```python
from build123d import *

# Parameters (mm, degrees)
SKETCH_1_R               = 10
EXTRUDE_1_DEPTH          = 4
SKETCH_3_R               = 3
CUT_EXTRUDE_1_DEPTH      = 15.696938457
SKETCH_5_R               = 1
CUT_EXTRUDE_2_DEPTH      = 15.696938457
PATTERN_CIRCULAR_1_COUNT = 8
SKETCH_6_R               = 3.5
SKETCH_6_R_2             = 3
EXTRUDE_3_DEPTH          = 0.5
FILLET_3_R               = 0.2
EXTRUDE_START            = -1.6
SKETCH_7_R               = 3.5
SKETCH_7_R_2             = 1.25
EXTRUDE_4_DEPTH          = 1.6


with BuildPart() as part:
    # Sketch 1 → Extrude 1 (new body)
    with BuildSketch(Plane(origin=(0, 0, 0), x_dir=(0, 0, -1), z_dir=(1, 0, 0))):
        Circle(SKETCH_1_R)
    extrude(amount=EXTRUDE_1_DEPTH)

    # Sketch 3 → Cut-Extrude 1 (cut, through all)
    with BuildSketch(Plane(origin=(4, 0, 0), x_dir=(0, 0, -1), z_dir=(1, 0, 0))):
        Circle(SKETCH_3_R)
    extrude(amount=-CUT_EXTRUDE_1_DEPTH, mode=Mode.SUBTRACT)

    # Sketch 5 → Cut-Extrude 2 (cut, through all)
    with BuildSketch(Plane.ZY):
        with Locations((0, 7)):
            Circle(SKETCH_5_R)
    cut_extrude_2 = extrude(amount=-CUT_EXTRUDE_2_DEPTH, mode=Mode.SUBTRACT)

    # Pattern Circular 1: Cut-Extrude 2 ×8 about axis
    pattern_circular_1_axis = Axis((0, 0, 0), (1, 0, 0))
    for i in range(1, PATTERN_CIRCULAR_1_COUNT):
        add(cut_extrude_2.rotate(pattern_circular_1_axis, i * 360 / PATTERN_CIRCULAR_1_COUNT), mode=Mode.SUBTRACT)

    # Sketch 6 → Extrude 3 (add)
    with BuildSketch(Plane.ZY):
        with Locations(Location((0, 0, 0), (0, 0, 180))):
            Circle(SKETCH_6_R)
        with Locations(Location((0, 0, 0), (0, 0, 180))):
            Circle(SKETCH_6_R_2, mode=Mode.SUBTRACT)
    extrude(amount=EXTRUDE_3_DEPTH)

    # Fillet 3
    fillet_3_edges = [part.edges().sort_by_distance(p)[0] for p in [
        (-0.5, 0, 3.5),
        (-0.5, 0, 3),
    ]]
    fillet(fillet_3_edges, radius=FILLET_3_R)

    # Sketch 7 → Extrude 4 (add)
    with BuildSketch(Plane.ZY.offset(EXTRUDE_START)):
        with Locations(Location((0, 0, 0), (0, 0, 180))):
            Circle(SKETCH_7_R)
        Circle(SKETCH_7_R_2, mode=Mode.SUBTRACT)
    extrude(amount=EXTRUDE_4_DEPTH)


solid = part.part
```
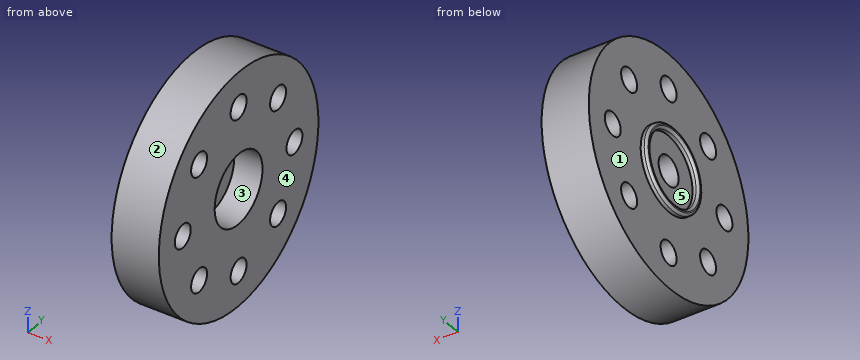
Could you check a few things on this model? Use its own coordinates, in mm. Face numbers are marked on the shaded views. A direction names the side the tool comes from. Round coordinates to 2 decimals unless told otherwise and drop trailing zeros. Loops run counter-clockwise (first coordinate to the right, second up) from the corner with the lowest first, then second, coordinate; pieces in that order, holes last.
Q1. Thinking about a two-plate mould opening in Y: for the marked faces 1, 2 and 3, which applies, pulls with the +Y half, pulls with the -Y half, needs draft (parallel to the pull), parting line crosses it, or undercut?
Q2. For P1, Ø3.5, axis at y = 0, z = 0, coming from the +X side; P2, Ø1.2, axis at y = -4.95, z = -4.95, coming from the -X side; P3, Ø3, axis at y = 7, z = 0, coming from the -X side; P4, Ø2, axis at x = 0.5, z = 3, coming from the -Y side, each with a flat end and sliding along its axis, tell me the tip position at first contact or that it passes through.
Q3. Please list where these lines run through material, in increasing order: L1, parallel to Y at x = 1.1, z = 0; L2, parallel to Y at x = 1.65, z = -5.75; L3, parallel to Z at x = 2.55, y = 4.75.
Q4. I want a section at B-B (x = 2.9). Give the number of separate pieces and of enclosed holes in the cut face, and give its area (3 significant figures).
Q5. I want a section at D-D (y = -5.25). Write out the boundary of the cut face in (x, z).
Q6. I want a section at A-A (z = 7). Write out the boundary of the cut face in (x, y).
Q7. On a 3-axis mill with a long thin cutter (end or side, diameter ignored), from which of +Z, -Z, +X, -X, +Y, -Y can I reach the whole of each face in a straight line? I mean the marked faces 4 and 5. Say none if no direction works.
Answer below:
1. face 1: needs draft
1. face 2: parting line crosses it
1. face 3: undercut
2. P1: stops at x = 1.6
2. P2: passes through
2. P3: stops at x = 0
2. P4: stops at y = -9.8
3. L1: y = -10 to -8, -6 to -1.25, 1.25 to 6, 8 to 10
3. L2: y = -8.18 to -5.55, -4.35 to 4.35, 5.55 to 8.18
3. L3: z = -8.8 to -5.93, -3.97 to 3.97, 5.93 to 8.8
4. separate pieces: 1
4. enclosed holes: 9
4. area: 261 mm2
5. outline: (0, -8.51) - (4, -8.51) - (4, -5.9) - (0, -5.9) - close; (0, -4) - (4, -4) - (4, 4) - (0, 4) - close; (0, 5.9) - (4, 5.9) - (4, 8.51) - (0, 8.51) - close
6. outline: (0, -7.14) - (4, -7.14) - (4, -1) - (0, -1) - close; (0, 1) - (4, 1) - (4, 7.14) - (0, 7.14) - close
7. face 4: +Z, -Z, +X, +Y, -Y
7. face 5: -X
